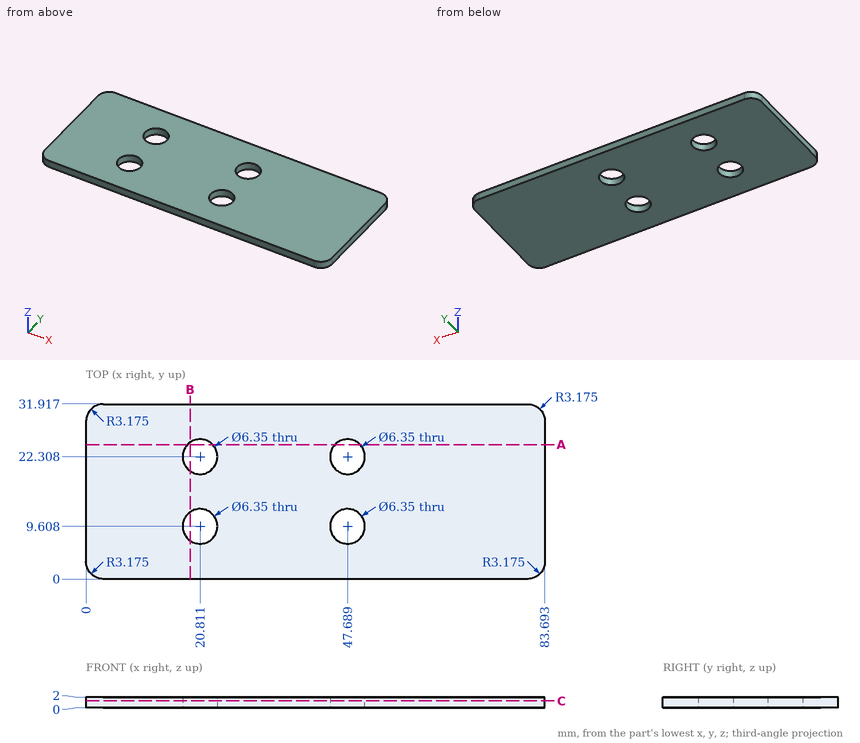
Here's the drawing with two shaded views (mm, measured from the low corner). I have some questions. Give positions to 0.01 mm unless a question says otherwise; leave off trailing zeros. Write each loop counter-clockwise with the first axis right and the second up, starting at its lowest first coordinate (ties: lowest second). Pieces come first, ordered by that corner, then holes. Notation, with made-up numbers: (65.5, 45.25) - (123.5, 45.25) arc R14 cw to (123.5, 57.25) - close; hole circle Ø1 at (42.25, -26). An arc over 180 degrees is marked (long way). One line per item, written item: value. Start each with the question number.
Item 1: I'm going to push a flat-ended pin straight in: pin 1 (5.5 mm diameter, centred on x = 20.81, y = 9.61, fed in from -Z). Where does the tip first touch, or does it pass through?
Item 2: Imagine slicing it at A-A, the plane y = 24.5. List the corners of the cut face in (x, z) for me.
Item 3: Imagine slicing it at C-C, the plane z = 1.3. Give the number of separate pieces and of enclosed holes in the cut face, and give its area (3 significant figures).
Item 4: Imagine slicing it at B-B, the plane x = 19. List the corners of the cut face in (y, z) for me.
Item 5: Please list where these lines run through material, in increasing order: line 1 (X direction, y = 22, z = 0.9); line 2 (X direction, y = 25, z = 1.4) (1 decimal); line 3 (Y direction, x = 50.5, z = 0.2) (1 decimal). Write a range as from..to.
Geometry says:
1. pin 1: through
2. outline: (0, 0) - (18.51, 0) - (18.51, 2) - (0, 2) - close; (23.11, 0) - (45.39, 0) - (45.39, 2) - (23.11, 2) - close; (49.99, 0) - (83.69, 0) - (83.69, 2) - (49.99, 2) - close
3. separate pieces: 1
3. enclosed holes: 4
3. area: 2,540 mm^2
4. outline: (0, 0) - (7, 0) - (7, 2) - (0, 2) - close; (12.22, 0) - (19.7, 0) - (19.7, 2) - (12.22, 2) - close; (24.92, 0) - (31.92, 0) - (31.92, 2) - (24.92, 2) - close
5. line 1: 0..17.65, 23.97..44.53, 50.85..83.69
5. line 2: 0..19.1, 22.5..46, 49.4..83.7
5. line 3: 0..8.1, 11.1..20.8, 23.8..31.9
